The listing builds one solid part. Answer for the finished solid, in the listing's coordinates (mm). Face numbers are marked on the shaded views. A direction names the side the tool comes from. Coordinates: 2 decimals unless noted, no trailing zeros. Write each loop counter-clockwise with the first axis right and the second up, starting at its lowest first coordinate (ties: lowest second). Pieces come first, ordered by that corner, then holes. Notation, with made-up numbers: M -27.5,61.25 L 5.5,61.25 A35 ccw 5.5,94.25 Z; hole C 71.25,38 d6. An arc over 180 degrees is marked long. Answer as CSV lines item,"result".
```python
from build123d import *

# Parameters (mm, degrees)
NECK_DEPTH   = 9.3726
HEADFILLET_R = 0.7874


with BuildPart() as part:
    # BodySke → BaseBody (revolve)
    with BuildSketch(Plane.XY, mode=Mode.PRIVATE) as basebody_sk:
        Polygon((0, 0), (0, 16.9164), (0.381, 16.9164), (1.231924038, 16.065475962), (3.429, 4.7625), (76.2, 4.7625), (76.2, 0), align=None)
    revolve(basebody_sk.sketch.rotate(Axis((-6.35, 0, 0), (1, 0, 0)), 90), axis=Axis((-6.35, 0, 0), (1, 0, 0)))

    # Sketch2 → Neck (add)
    with BuildSketch(Plane(origin=(0, 0, 0), x_dir=(0, 0.6946583704589985, -0.7193398003386501), z_dir=(1, 0, 0))):
        with BuildLine():
            Line((3.7084, -4.9022), (-3.7084, -4.9022))
            ThreePointArc((-3.7084, -4.9022), (-4.552544075, -4.552544075), (-4.9022, -3.7084))
            Line((-4.9022, -3.7084), (-4.9022, 3.7084))
            ThreePointArc((-4.9022, 3.7084), (-4.552544075, 4.552544075), (-3.7084, 4.9022))
            Line((-3.7084, 4.9022), (3.7084, 4.9022))
            ThreePointArc((3.7084, 4.9022), (4.552544075, 4.552544075), (4.9022, 3.7084))
            Line((4.9022, 3.7084), (4.9022, -3.7084))
            ThreePointArc((4.9022, -3.7084), (4.552544075, -4.552544075), (3.7084, -4.9022))
        make_face()
    extrude(amount=NECK_DEPTH)

    # Sketch3 → NeckChamfer (revolve, cut)
    with BuildSketch(Plane.XY, mode=Mode.PRIVATE) as neckchamfer_sk:
        Polygon((2.713017566, 29.6164), (9.3726, 4.7625), (9.6266, 4.7625), (9.6266, 29.6164), align=None)
    revolve(neckchamfer_sk.sketch.rotate(Axis((0, 0, 0), (1, 0, 0)), 90), axis=Axis((0, 0, 0), (1, 0, 0)), mode=Mode.SUBTRACT)

    # HeadFillet
    headfillet_edges = [part.edges().sort_by_distance(p)[0] for p in [
        (3.401845071, 3.405354264, -3.526347569),
        (3.103263392, -0.112363299, -6.437288995),
        (3.401845071, -3.526347569, -3.405354264),
        (3.103263392, -6.437288995, 0.112363299),
        (3.401845071, -3.405354264, 3.526347569),
        (3.121431163, -0.398458833, 6.332280366),
        (3.401845071, 3.526347569, 3.405354264),
        (3.103263392, 6.437288995, -0.112363299),
    ]]
    fillet(headfillet_edges, radius=HEADFILLET_R)


solid = part.part
```
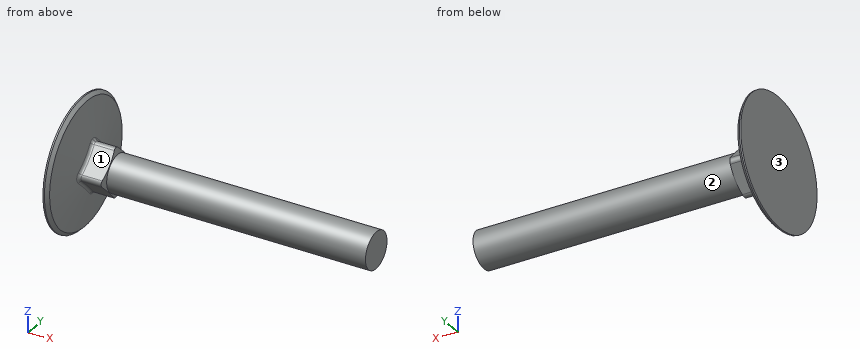
Q1. Find section A-A (x = 64.5). Give the vertices of the cut face in (y, z) (1 decimal), and give its area (3 significant figures).
Output:
outline,"C 0,0 d9.5"
area,"71.3 mm2"
Q2. Flat-ended cylindrical pins translate along their axes: pin 1 Ø5 at (x, y) = (15.5, 5) entering from -Z; pin 2 Ø5 at (x, z) = (33, 0.5) entering from -Y; pin 3 Ø5 at (x, y) = (53, 3.5) entering from -Z; pin 4 Ø8 at (y, z) = (-4.5, 7) entering from +X. Find the tip coordinate at first contact, or state that the pin passes through.
Output:
pin 1,"z = -4.05"
pin 2,"y = -4.76"
pin 3,"z = -4.66"
pin 4,"x = 76.2"
Q3. Straight lines are drawn through the part: line 1 (X direction, y = 3, z = -6.5); line 2 (X direction, y = -15, z = -6.5); line 3 (Y direction, x = 70.5, z = -4). For each, find the intervals that lie inside material, in ascending order.
Output:
line 1,"0 to 2.96"
line 2,"0 to 0.95"
line 3,"-2.58 to 2.58"
Q4. For the marked faces 1, 2 and 3, determine the directions among +Z, -Z, +X, -X, +Y, -Y from which every point of the face is accessible in a straight line to the end or side of a thin tool.
Output:
face 1,"+Z, +X, -Y"
face 2,"+X"
face 3,"+Z, -Z, -X, +Y, -Y"
